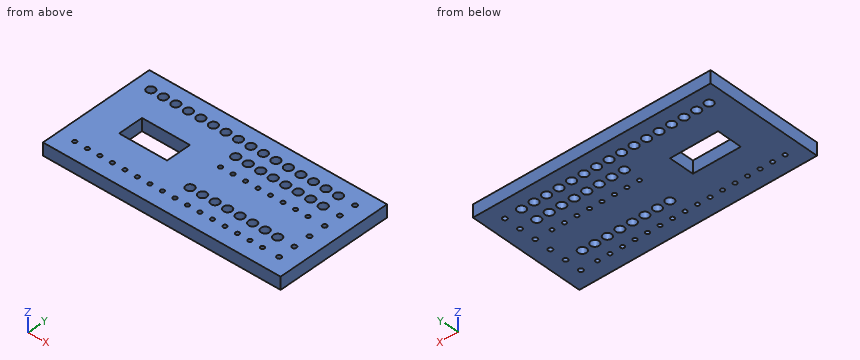
from build123d import *

# Parameters (mm, degrees)
SKETCH1_W           = 361.95
SKETCH1_H           = 177.8
SKETCH1_R           = 6.35
SKETCH1_R_2         = 3
SKETCH1_R_3         = 3.4
SKETCH1_W_2         = 73.025
SKETCH1_H_2         = 38.1
BOSS_EXTRUDE1_DEPTH = 19.05


with BuildPart() as part:
    # Sketch1 → Boss-Extrude1 (new body)
    with BuildSketch(Plane.XY):
        with Locations((106.3625, -11.579089164)):
            Rectangle(SKETCH1_W, SKETCH1_H)
        with Locations((-49.2125, 51.920910836)):
            Circle(SKETCH1_R, mode=Mode.SUBTRACT)
        with Locations((-30.1625, 51.920910836)):
            Circle(SKETCH1_R, mode=Mode.SUBTRACT)
        with Locations((-11.1125, 51.920910836)):
            Circle(SKETCH1_R, mode=Mode.SUBTRACT)
        with Locations((7.9375, 51.920910836)):
            Circle(SKETCH1_R, mode=Mode.SUBTRACT)
        with Locations((26.9875, 51.920910836)):
            Circle(SKETCH1_R, mode=Mode.SUBTRACT)
        with Locations((46.0375, 51.920910836)):
            Circle(SKETCH1_R, mode=Mode.SUBTRACT)
        with Locations((65.0875, 51.920910836)):
            Circle(SKETCH1_R, mode=Mode.SUBTRACT)
        with Locations((84.1375, 51.920910836)):
            Circle(SKETCH1_R, mode=Mode.SUBTRACT)
        with Locations((103.1875, 51.920910836)):
            Circle(SKETCH1_R, mode=Mode.SUBTRACT)
        with Locations((122.2375, 51.920910836)):
            Circle(SKETCH1_R, mode=Mode.SUBTRACT)
        with Locations((141.2875, 51.920910836)):
            Circle(SKETCH1_R, mode=Mode.SUBTRACT)
        with Locations((160.3375, 51.920910836)):
            Circle(SKETCH1_R, mode=Mode.SUBTRACT)
        with Locations((179.3875, 51.920910836)):
            Circle(SKETCH1_R, mode=Mode.SUBTRACT)
        with Locations((198.4375, 51.920910836)):
            Circle(SKETCH1_R, mode=Mode.SUBTRACT)
        with Locations((217.4875, 51.920910836)):
            Circle(SKETCH1_R, mode=Mode.SUBTRACT)
        with Locations((236.5375, 51.920910836)):
            Circle(SKETCH1_R, mode=Mode.SUBTRACT)
        with Locations((103.1875, 26.520910836)):
            Circle(SKETCH1_R, mode=Mode.SUBTRACT)
        with Locations((122.2375, 26.520910836)):
            Circle(SKETCH1_R, mode=Mode.SUBTRACT)
        with Locations((141.2875, 26.520910836)):
            Circle(SKETCH1_R, mode=Mode.SUBTRACT)
        with Locations((160.3375, 26.520910836)):
            Circle(SKETCH1_R, mode=Mode.SUBTRACT)
        with Locations((179.3875, 26.520910836)):
            Circle(SKETCH1_R, mode=Mode.SUBTRACT)
        with Locations((198.4375, 26.520910836)):
            Circle(SKETCH1_R, mode=Mode.SUBTRACT)
        with Locations((217.4875, 26.520910836)):
            Circle(SKETCH1_R, mode=Mode.SUBTRACT)
        with Locations((236.5375, 26.520910836)):
            Circle(SKETCH1_R, mode=Mode.SUBTRACT)
        with Locations((103.1875, -49.679089164)):
            Circle(SKETCH1_R, mode=Mode.SUBTRACT)
        with Locations((122.2375, -49.679089164)):
            Circle(SKETCH1_R, mode=Mode.SUBTRACT)
        with Locations((141.2875, -49.679089164)):
            Circle(SKETCH1_R, mode=Mode.SUBTRACT)
        with Locations((160.3375, -49.679089164)):
            Circle(SKETCH1_R, mode=Mode.SUBTRACT)
        with Locations((179.3875, -49.679089164)):
            Circle(SKETCH1_R, mode=Mode.SUBTRACT)
        with Locations((198.4375, -49.679089164)):
            Circle(SKETCH1_R, mode=Mode.SUBTRACT)
        with Locations((217.4875, -49.679089164)):
            Circle(SKETCH1_R, mode=Mode.SUBTRACT)
        with Locations((236.5375, -49.679089164)):
            Circle(SKETCH1_R, mode=Mode.SUBTRACT)
        with Locations((103.1875, 1.120910836)):
            Circle(SKETCH1_R_2, mode=Mode.SUBTRACT)
        with Locations((122.2375, 1.120910836)):
            Circle(SKETCH1_R_2, mode=Mode.SUBTRACT)
        with Locations((141.2875, 1.120910836)):
            Circle(SKETCH1_R_2, mode=Mode.SUBTRACT)
        with Locations((160.3375, 1.120910836)):
            Circle(SKETCH1_R_2, mode=Mode.SUBTRACT)
        with Locations((179.3875, 1.120910836)):
            Circle(SKETCH1_R_2, mode=Mode.SUBTRACT)
        with Locations((198.4375, 1.120910836)):
            Circle(SKETCH1_R_2, mode=Mode.SUBTRACT)
        with Locations((217.4875, 1.120910836)):
            Circle(SKETCH1_R_2, mode=Mode.SUBTRACT)
        with Locations((236.5375, 1.120910836)):
            Circle(SKETCH1_R_2, mode=Mode.SUBTRACT)
        with Locations((-49.2125, -75.079089164)):
            Circle(SKETCH1_R_2, mode=Mode.SUBTRACT)
        with Locations((-30.1625, -75.079089164)):
            Circle(SKETCH1_R_2, mode=Mode.SUBTRACT)
        with Locations((-11.1125, -75.079089164)):
            Circle(SKETCH1_R_2, mode=Mode.SUBTRACT)
        with Locations((7.9375, -75.079089164)):
            Circle(SKETCH1_R_2, mode=Mode.SUBTRACT)
        with Locations((26.9875, -75.079089164)):
            Circle(SKETCH1_R_2, mode=Mode.SUBTRACT)
        with Locations((46.0375, -75.079089164)):
            Circle(SKETCH1_R_2, mode=Mode.SUBTRACT)
        with Locations((65.0875, -75.079089164)):
            Circle(SKETCH1_R_2, mode=Mode.SUBTRACT)
        with Locations((84.1375, -75.079089164)):
            Circle(SKETCH1_R_2, mode=Mode.SUBTRACT)
        with Locations((103.1875, -75.079089164)):
            Circle(SKETCH1_R_2, mode=Mode.SUBTRACT)
        with Locations((122.2375, -75.079089164)):
            Circle(SKETCH1_R_2, mode=Mode.SUBTRACT)
        with Locations((141.2875, -75.079089164)):
            Circle(SKETCH1_R_2, mode=Mode.SUBTRACT)
        with Locations((160.3375, -75.079089164)):
            Circle(SKETCH1_R_2, mode=Mode.SUBTRACT)
        with Locations((179.3875, -75.079089164)):
            Circle(SKETCH1_R_2, mode=Mode.SUBTRACT)
        with Locations((198.4375, -75.079089164)):
            Circle(SKETCH1_R_2, mode=Mode.SUBTRACT)
        with Locations((217.4875, -75.079089164)):
            Circle(SKETCH1_R_2, mode=Mode.SUBTRACT)
        with Locations((236.5375, -75.079089164)):
            Circle(SKETCH1_R_2, mode=Mode.SUBTRACT)
        with Locations((261.9375, 51.920910836)):
            Circle(SKETCH1_R_3, mode=Mode.SUBTRACT)
        with Locations((261.9375, 26.520910836)):
            Circle(SKETCH1_R_3, mode=Mode.SUBTRACT)
        with Locations((261.9375, -24.279089164)):
            Circle(SKETCH1_R_3, mode=Mode.SUBTRACT)
        with Locations((261.9375, -75.079089164)):
            Circle(SKETCH1_R_3, mode=Mode.SUBTRACT)
        with Locations((261.9375, -49.679089164)):
            Circle(SKETCH1_R_3, mode=Mode.SUBTRACT)
        with Locations((261.9375, 1.120910836)):
            Circle(SKETCH1_R_3, mode=Mode.SUBTRACT)
        with Locations((14.2875, -11.579089164)):
            Rectangle(SKETCH1_W_2, SKETCH1_H_2, mode=Mode.SUBTRACT)
    extrude(amount=BOSS_EXTRUDE1_DEPTH)


solid = part.part
Build history of the part. All positions in model axes, mm. Coordinates: 2 decimals unless noted, no trailing zeros.
(1) Cut at A-A on z = 5.5. State how many separate pieces and enclosed holes the cut face has, and give its area (3 significant figures).
(2) Drill centre lines: line 1 (X direction, y = -25, z = 8.25) (1 decimal); line 2 (X direction, y = -11, z = 2) (1 decimal); line 3 (Y direction, x = 50, z = 4.75). Where is each one in solid material? Low to high.
(3) Pin check, flat tip, straight feed: pin 1 Ø11.5 at (x, y) = (26.99, 51.92) entering from -Z. Stop position of the tip, or through.
Working result:
1. separate pieces: 1
1. enclosed holes: 63
1. area: 56,600 mm2
2. line 1: x = -74.6 to -22.2, 50.8 to 258.6, 265.3 to 287.3
2. line 2: x = -74.6 to -22.2, 50.8 to 287.3
2. line 3: y = -100.48 to -30.63, 7.47 to 46.96, 56.88 to 77.32
3. pin 1: passes through
